Part model, mm, in its own coordinate system. A direction names the side the tool comes from. Coordinates: 2 decimals unless noted, no trailing zeros. Order: outer loops, then holes, each group sorted by start corner. A loop starts at its lowest first (then second) coordinate and runs counter-clockwise, first axis right, second up. Notation, with made-up numbers: (37, 12.5) - (72, 12.5) arc R11 ccw to (72, 17.5) - close; hole circle Ø7 at (89, -3). An arc over 180 degrees is marked (long way). Use a Markdown table: item, result. Add a question column.
1) Two-plate mould, pull along X, no slides. Class faces 4 (the face through (0, 19, 5)), 5 (the face through (-26, -22, 3)), 6 (the face through (0, 17, 5)), 7 (the face through (-19, -11, 5)): +X half, -X half, draft (parallel to the pull), parting line (faces both ways), or undercut.
2) Saw through at B-B on y = -3. List the corners of the cut face in (x, z), then the cut area to 3 significant figures.
3) Wall check: L1, parallel to Z at x = -24, y = -23.15; L2, parallel to X at y = -3, z = 1.25; L3, parallel to Y at x = -24.5, z = 2.5. Give the ranges that are in metal, low to high. Write a range as [from, to].
4) Tool access for faces 1 (the face through (19, -11, 5)), 2 (the face through (17.3, -4.5, 10)), 3 (the face through (17, -13, 5)): list every direction of +Z, -Z, +X, -X, +Y, -Y with a clear straight run to the whole face (end or side of a thin tool).
5) Saw through at D-D on x = 9.5. List the corners of the cut face in (y, z).
6) Drop flat-ended pins along their axis: P1, Ø1.5, axis at y = 11, z = 6.5, coming from the -X side; P2, Ø3, axis at y = 12.5, z = 5, coming from the +X side; P3, Ø5, axis at y = -14, z = 7, coming from the +X side. Give the stop position or say it passes through.
7) Saw through at C-C on x = 0. List the corners of the cut face in (y, z).
8) Saw through at A-A on x = -24. List the corners of the cut face in (y, z).
```python
from build123d import *

# Parameters (mm, degrees)
BOSS_EXTRUDE1_DEPTH = 10
SKETCH2_R           = 2.534927605
SKETCH2_R_2         = 2.5
CUT_EXTRUDE1_DEPTH  = 10


with BuildPart() as part:
    # Sketch1 → Boss-Extrude1 (new body)
    with BuildSketch(Plane.XY):
        with BuildLine():
            Line((-17, 0), (-17, -24))
            Line((-17, -24), (-17, -25))
            Line((-17, -25), (-29, -25))
            Line((-29, -25), (-29, -22))
            Line((-29, -22), (-19, -22))
            Line((-19, -22), (-19, 0))
            ThreePointArc((-19, 0), (0, 19), (19, 0))
            Line((19, 0), (19, -22))
            Line((19, -22), (29, -22))
            Line((29, -22), (29, -25))
            Line((29, -25), (17, -25))
            Line((17, -25), (17, -24))
            Line((17, -24), (17, 0))
            ThreePointArc((17, 0), (0, 17), (-17, 0))
        make_face()
    extrude(amount=BOSS_EXTRUDE1_DEPTH)

    # Sketch2 → Cut-Extrude1 (cut)
    with BuildSketch(Plane(origin=(0, -22, 0), x_dir=(1, 0, 0), z_dir=(0, 1, 0))):
        with Locations((-24, -5.101003531)):
            Circle(SKETCH2_R)
        with Locations((24.304859837, -5.101003531)):
            Circle(SKETCH2_R_2)
    extrude(amount=-CUT_EXTRUDE1_DEPTH, mode=Mode.SUBTRACT)


solid = part.part
```
Results are:
| question | item | result |
|---|---|---|
| 1 | face 4 | parting line |
| 1 | face 5 | draft |
| 1 | face 6 | undercut |
| 1 | face 7 | -X half |
| 2 | outline | (-19, 0) - (-17, 0) - (-17, 10) - (-19, 10) - close; (17, 0) - (19, 0) - (19, 10) - (17, 10) - close |
| 2 | area | 40.0 mm2 |
| 3 | L1 | [0, 2.57], [7.64, 10] |
| 3 | L2 | [-19, -17], [17, 19] |
| 3 | L3 | [-25, -22] |
| 4 | face 1 | +Z, -Z, +X, +Y |
| 4 | face 2 | +Z, +X, -X, +Y, -Y |
| 4 | face 3 | +Z, -Z, -Y |
| 5 | outline | (14.1, 0) - (16.45, 0) - (16.45, 10) - (14.1, 10) - close |
| 6 | P1 | x = -16 |
| 6 | P2 | x = 15.49 |
| 6 | P3 | x = 19 |
| 7 | outline | (17, 0) - (19, 0) - (19, 10) - (17, 10) - close |
| 8 | outline | (-25, 0) - (-22, 0) - (-22, 2.57) - (-25, 2.57) - close; (-25, 7.64) - (-22, 7.64) - (-22, 10) - (-25, 10) - close |
